Could you check a few things on this model? Use its own coordinates, in mm. A direction names the side the tool comes from. Round coordinates to 2 decimals unless told otherwise and drop trailing zeros. Write each loop counter-clockwise with the first axis right and the second up, starting at its lowest first coordinate (ties: lowest second). Pieces come first, ordered by that corner, then holes. Notation, with made-up numbers: (39, 65) - (89, 65) arc R29 cw to (89, 95) - close; hole circle Ø10 at (39.25, 6). An arc over 180 degrees is marked (long way). Write each question's results on one line, items separated by ' | '. Start each with the question number.
(1) For P1, Ø1.3, axis at y = 32.5, z = 8.5, coming from the -X side; P2, Ø1.8, axis at x = 3, z = 8.5, coming from the +Y side; P3, Ø0.8, axis at y = -20, z = 8, coming from the +X side, each with a flat end and sliding along its axis, tell me the tip position at first contact or that it passes through.
(2) Imagine slicing it at A-A on x = -16. Write out the boundary of the cut face in (y, z), then the cut area to 3 significant figures.
(3) On a 3-axis mill with a long thin cutter (end or side, diameter ignored), from which of +Z, -Z, +X, -X, +Y, -Y can I reach the whole of each face in a straight line? I mean faces 4 (the flat face through (0, -93, 4)), 5 (the flat face through (-30, 1, 7.4)). Say none if no direction works.
(4) Imagine slicing it at B-B on y = 59. Write out the boundary of the cut face in (x, z).
(5) Please list where these lines run through material, in increasing order: line 1 (Y direction, x = 20.5, z = 3); line 2 (X direction, y = 76.5, z = 3.5); line 3 (Z direction, x = 7, y = -84). Write a range as [from, to].
(6) Thinking about a two-plate mould opening in X: for faces 1 (the cylindrical face through (-20.695, -75.013, 3.752)), 2 (the flat face through (33.5, -1, 4)), 3 (the flat face through (0, 1, 9)), which applies, +X half, -X half, draft (parallel to the pull), parting line (faces both ways), or undercut?
(7) Imagine slicing it at C-C on y = 80. Write out the boundary of the cut face in (x, z).
Autodesk Inventor part; units mm, degrees
ref_plane "YZ Plane" through (0, 0, 0) normal (1, 0, 0) x (0, 1, 0)
ref_plane "XZ Plane" through (0, 0, 0) normal (0, 1, 0) x (-1, 0, 0)
ref_plane "XY Plane" through (0, 0, 0) normal (0, 0, 1) x (1, 0, 0)
sketch "Sketch1" plane through (0, 0, 0) normal (0, 0, 1) x (1, 0, 0)
  line L0 (-33.5, -93) -> (33.5, -93)
  line L1 (33.5, -93) -> (33.5, 93)
  line L2 (33.5, 93) -> (-33.5, 93)
  line L3 (-33.5, 93) -> (-33.5, -93)
  line L4 (-33.5, -93) -> (33.5, 93) construction
  line L5 (33.5, -93) -> (-33.5, 93) construction
  point P0 (0, 0)
  dimension "d0" = 67
  dimension "d1" = 186
extrude "Extrusion1" add sketch "Sketch1" along normal blind 7.4
sketch "Sketch2" plane through (0, 0, 7.4) normal (0, 0, 1) x (1, 0, 0)
  line L0 (24, 71.3) -> (-24, 71.3)
  line L1 (-24, 71.3) -> (-24, -71.3)
  line L2 (-24, -71.3) -> (24, -71.3)
  line L3 (24, -71.3) -> (24, 71.3)
  line L4 (24, 71.3) -> (-24, -71.3) construction
  line L5 (-24, 71.3) -> (24, -71.3) construction
  point P0 (0, 0)
  dimension "d4" = 48
  dimension "d5" = 142.6
extrude "Extrusion2" add sketch "Sketch2" along normal blind 1.6
fillet "Fillet1" radius 2 8 edges at (24, 71.3, 8.2) (-24, 71.3, 8.2) (-24, -71.3, 8.2) (24, -71.3, 8.2) (-33.5, 93, 3.7) (33.5, 93, 3.7) (-33.5, -93, 3.7) (33.5, -93, 3.7)
sketch "Sketch3" plane through (0, 0, 9) normal (0, 0, 1) x (1, 0, 0)
  circle A0 centre (-20.5, -76.5) radius 1.5
  line L0 (-46.9, 0) -> (46.9, 0) construction
  line L1 (0, -130.2) -> (0, 130.2) construction
  circle A1 centre (-20.5, 76.5) radius 1.5
  circle A2 centre (20.5, -76.5) radius 1.5
  circle A3 centre (20.5, 76.5) radius 1.5
  point P0 (0, 0)
  dimension "d9" = 3
  dimension "d10" = 41
  dimension "d11" = 153
extrude "Extrusion3" cut sketch "Sketch3" against normal through all
properties part number "PanelJig"
Response:
1) P1: x = -24 | P2: y = 71.3 | P3: x = 24
2) outline: (-93, 0) - (93, 0) - (93, 7.4) - (71.3, 7.4) - (71.3, 9) - (-71.3, 9) - (-71.3, 7.4) - (-93, 7.4) - close | area: 1,600 mm²
3) face 4: +Z, -Z, +X, -X, -Y | face 5: +Z
4) outline: (-33.5, 0) - (33.5, 0) - (33.5, 7.4) - (24, 7.4) - (24, 9) - (-24, 9) - (-24, 7.4) - (-33.5, 7.4) - close
5) line 1: [-93, -78], [-75, 75], [78, 93] | line 2: [-33.5, -22], [-19, 19], [22, 33.5] | line 3: [0, 7.4]
6) face 1: undercut | face 2: +X half | face 3: draft
7) outline: (-33.5, 0) - (33.5, 0) - (33.5, 7.4) - (-33.5, 7.4) - close
